Verification items for the finished model (mm, model axes). A direction names the side the tool comes from. Coordinates: 2 decimals unless noted, no trailing zeros. Write each loop counter-clockwise with the first axis right and the second up, starting at its lowest first coordinate (ties: lowest second). Pieces come first, ordered by that corner, then holes. Notation, with made-up numbers: (64, 14.5) -> (112, 14.5) arc R20 ccw to (112, 31.5) -> close; hole circle Ø1 at (7.25, 15.25). An arc over 180 degrees is marked (long way). Use CSV: the item, a comma, the result in double quotes.
```python
from build123d import *

# Parameters (mm, degrees)
F0_W     = 3
F0_H     = 5
F0_W_2   = 1.5
F1_DEPTH = 3


with BuildPart() as f1:
    # F0 (on Right) → F1 (new body)
    with BuildSketch(Plane.YZ):
        Polygon((1.5, 5), (1.5, 0), (4.5, 0), (4.5, -2), (11.5, -2), (11.5, 0), (14.5, 0), (14.5, 5), (14.5, 10), (11.5, 10), (1.5, 10), align=None)
        with Locations((16, 7.5)):
            Rectangle(F0_W, F0_H)
        Polygon((20.5, 10), (17.5, 10), (17.5, 5), (17.5, 0), (30.5, 0), (30.5, 5), (30.5, 10), align=None)
        with Locations((32, 7.5)):
            Rectangle(F0_W, F0_H)
        Polygon((33.5, 5), (33.5, 0), (36.5, 0), (36.5, -2), (43.5, -2), (43.5, 0), (48, 0), (52.5, 0), (52.5, -2), (59.5, -2), (59.5, 0), (62.5, 0), (62.5, 5), (62.5, 10), (33.5, 10), align=None)
        with Locations((64, 7.5)):
            Rectangle(F0_W, F0_H)
        Polygon((78.5, 10), (65.5, 10), (65.5, 5), (65.5, 0), (78.5, 0), (78.5, 5), align=None)
        with Locations((80, 7.5)):
            Rectangle(F0_W, F0_H)
        Polygon((110.5, 10), (81.5, 10), (81.5, 5), (81.5, 0), (84.5, 0), (84.5, -2), (91.5, -2), (91.5, 0), (96, 0), (100.5, 0), (100.5, -2), (107.5, -2), (107.5, 0), (110.5, 0), (110.5, 5), align=None)
        with Locations((112, 7.5)):
            Rectangle(F0_W, F0_H)
        Polygon((126.5, 10), (113.5, 10), (113.5, 5), (113.5, 0), (126.5, 0), (126.5, 5), align=None)
        with Locations((128, 7.5)):
            Rectangle(F0_W, F0_H)
        Polygon((158.5, 10), (129.5, 10), (129.5, 5), (129.5, 0), (132.5, 0), (132.5, -2), (139.5, -2), (139.5, 0), (144, 0), (148.5, 0), (148.5, -2), (155.5, -2), (155.5, 0), (158.5, 0), (158.5, 5), align=None)
        with Locations((160, 7.5)):
            Rectangle(F0_W, F0_H)
        Polygon((171.5, 10), (161.5, 10), (161.5, 5), (161.5, 0), (174.5, 0), (174.5, 5), (174.5, 10), align=None)
        with Locations((176, 7.5)):
            Rectangle(F0_W, F0_H)
        Polygon((180.5, 10), (177.5, 10), (177.5, 5), (177.5, 0), (180.5, 0), (180.5, -2), (187.5, -2), (187.5, 0), (190.5, 0), (190.5, 5), (190.5, 10), align=None)
        with Locations((0.75, 7.5)):
            Rectangle(F0_W_2, F0_H)
        with Locations((191.25, 7.5)):
            Rectangle(F0_W_2, F0_H)
        with Locations((192.75, 7.5)):
            Rectangle(F0_W_2, F0_H)
        with Locations((-0.75, 7.5)):
            Rectangle(F0_W_2, F0_H)
    extrude(amount=F1_DEPTH)


solid = f1.part
```
1) Scan line: L1, parallel to Z at x = 1.3, y = 78. Record every from-to range of solid material in increasing order.
Return value:
L1,"0 to 10"
2) Cross-section at A-A (z = 3). Give the number of separate pieces and of enclosed holes in the cut face, plus the area to 3 significant figures.
Return value:
separate pieces,"9"
enclosed holes,"0"
area,"495 mm2"
3) Gauge pin test, flat ends, axial feed: pin 1 (1.5 mm diameter, centred on x = 1, y = 128, fed in from -Z); pin 2 (0.9 mm diameter, centred on x = 1.5, z = 3, fed in from -Y); pin 3 (0.6 mm diameter, centred on x = 2, z = -1, fed in from -Y). Record the tip position at first contact, or that the pin passes through.
Return value:
pin 1,"z = 5"
pin 2,"y = 1.5"
pin 3,"y = 4.5"
4) Set-up check for faces 1 (the flat face through (1, 104, -2)), 2 (the flat face through (1, 113.5, 3)), 3 (the flat face through (1, 190.5, 2)): record each of +Z, -Z, +X, -X, +Y, -Y from which the full face is reachable in a straight line by a thin tool's end or side.
Return value:
face 1,"-Z, +X, -X, +Y, -Y"
face 2,"-Z, +X, -X"
face 3,"-Z, +X, -X, +Y"
5) Mould release check, pull along Y, two halves, no side actions. Record for faces 4 (the flat face through (1, 193.5, 7)), 5 (the flat face through (0, 95, 4)), 6 (the flat face through (1, 157, 0)): released by +Y, released by -Y, zero draft, split by the parting line, or undercut.
Return value:
face 4,"released by +Y"
face 5,"zero draft"
face 6,"undercut"
6) Cross-section at B-B (y = 74). Record the boundary of the cut face in (x, z), plus the area to 3 significant figures.
Return value:
outline,"(0, 0) -> (3, 0) -> (3, 10) -> (0, 10) -> close"
area,"30.0 mm2"
